```python
from build123d import *

# Parameters (mm, degrees)
F0_R     = 31.75
F1_DEPTH = 25.4
F2_SIZE  = 22.86
F5_T     = -1.27


# Not quite as in the source:
# - a fillet or chamfer that OpenCascade refuses, or shapes differently, is made with other operations: its cross-section is extruded or revolved along the edge and cut away or added
# - a feature of the source that left no trace in its solid (it failed there, or was rolled back) is left out
# - a shell that OpenCascade refuses in one call is made with other operations: the cavity is built on its own and cut out


with BuildPart() as f1:
    # F0 (on Front) → F1 (new body)
    with BuildSketch(Plane.XZ):
        Circle(F0_R)
    extrude(amount=F1_DEPTH)

    # F2
    f2_edges = [f1.edges().sort_by_distance(p)[0] for p in [
        (-31.75, -25.4, 0),
    ]]
    chamfer(f2_edges, length=F2_SIZE)

    # F4: fillet of radius 5.08 on 2 edges, made by hand

    # F4_s1 → F4_t2 (revolve, cut)
    with BuildSketch(Plane.XY):
        with BuildLine():
            ThreePointArc((31.75, -0.4357951031), (31.3633080252, -2.3798269396), (30.2621024484, -4.0278975516))
            Line((30.2621024484, -4.0278975516), (31.75, -2.54))
            Line((31.75, -2.54), (31.75, -0.4357951031))
        make_face()
    revolve(axis=Axis((0, -2.54, 0), (0, -1, 0)), mode=Mode.SUBTRACT)

    # F4_s3 → F4_t4 (revolve, cut)
    with BuildSketch(Plane.XY):
        with BuildLine():
            ThreePointArc((31.75, -0.4357951031), (30.7435201994, -0.1101428151), (29.691417751, 0))
            Line((29.691417751, 0), (31.75, 0))
            Line((31.75, 0), (31.75, -0.4357951031))
        make_face()
    revolve(axis=Axis((0, 0, 0), (0, -1, 0)), mode=Mode.SUBTRACT)

    # F5: a shell. OpenCascade refuses it in one call, so the cavity is built on its own and cut out:
    # the body offset inwards by the wall thickness, plus a prism from it out through each open face.
    f5_core = offset(f1.part, amount=F5_T, mode=Mode.PRIVATE)
    f5_exits = [f5_core.faces().sort_by_distance(p)[0] for p in [
        (0, -1.27, 0),
    ]]
    add(f5_core, mode=Mode.SUBTRACT)
    extrude(f5_exits, amount=-F5_T, mode=Mode.SUBTRACT)


solid = f1.part
```
Input: part model. Units: mm. Frame: model coordinates. Coordinates: 2 decimals unless noted, no trailing zeros. Write each loop counter-clockwise with the first axis right and the second up, starting at its lowest first coordinate (ties: lowest second). Pieces come first, ordered by that corner, then holes.
1) Section C-C on y = -14. Output: boundary loops of the cut face in (x, z).
2) Material intervals for line 1 along Z through (x, y) = (0, -0.6); line 2 along X through (y, z) = (-1.75, 14); line 3 along Z through (x, y) = (1.5, -9), sorted ascending.
3) Section D-D on y = -7.75. Output: boundary loops of the cut face in (x, z), and give its area (3 significant figures).
4) Section B-B on x = 0. Output: boundary loops of the cut face in (y, z).
5) Section A-A on z = 0. Output: boundary loops of the cut face in (x, y), and give its area (3 significant figures).
6) Mould query, pull axis Z, two halves, no side actions, for faces 1 (the conical face through (-2.152, -24.362, -9.692)), 2 (the flat face through (0, -24.13, 0)), 3 (the flat face through (0, -25.4, 0)). Classes: pulls with the +Z half, pulls with the -Z half, needs draft (parallel to the pull), parting line crosses it, or undercut.
7) Pin query (flat end, axial travel): pin 1 Ø13.5 at (x, z) = (3, -0.5) entering from +Y; pin 2 Ø2 at (y, z) = (-6, -15.5) entering from -X; pin 3 Ø6 at (x, z) = (15, -14.5) entering from -Y. Return the tip coordinate at first contact, or that it passes through.
Check result:
1. outline: circle Ø40.58 at (0, 0); hole circle Ø36.99 at (0, 0)
2. line 1: z = -31.75 to -29.69, 29.69 to 31.75
2. line 2: x = -28.3 to -26.81, 26.81 to 28.3
2. line 3: z = -25.25 to -23.45, 23.45 to 25.25
3. outline: circle Ø53.08 at (0, 0); hole circle Ø49.49 at (0, 0)
3. area: 289 mm2
4. outline: (-25.4, -8.89) - (-4.03, -30.26) arc R5.08 ccw to (-0.44, -31.75) arc R5.08 ccw to (0, -29.69) - (-1.27, -29.69) arc R3.81 cw to (-1.33, -30.37) arc R3.81 cw to (-3.13, -29.36) - (-24.13, -8.36) - (-24.13, 8.36) - (-3.13, 29.36) arc R3.81 cw to (-1.33, 30.37) arc R3.81 cw to (-1.27, 29.69) - (0, 29.69) arc R5.08 ccw to (-0.44, 31.75) arc R5.08 ccw to (-4.03, 30.26) - (-25.4, 8.89) - close
5. outline: (-31.75, -0.44) arc R5.08 ccw to (-30.26, -4.03) - (-8.89, -25.4) - (8.89, -25.4) - (30.26, -4.03) arc R5.08 ccw to (31.75, -0.44) arc R5.08 ccw to (29.69, 0) - (29.69, -1.27) arc R3.81 cw to (30.37, -1.33) arc R3.81 cw to (29.36, -3.13) - (8.36, -24.13) - (-8.36, -24.13) - (-29.36, -3.13) arc R3.81 cw to (-30.37, -1.33) arc R3.81 cw to (-29.69, -1.27) - (-29.69, 0) arc R5.08 ccw to start
5. area: 109 mm2
6. face 1: parting line crosses it
6. face 2: undercut
6. face 3: needs draft
7. pin 1: stops at y = -22.7
7. pin 2: stops at x = -25
7. pin 3: stops at y = -16.43
